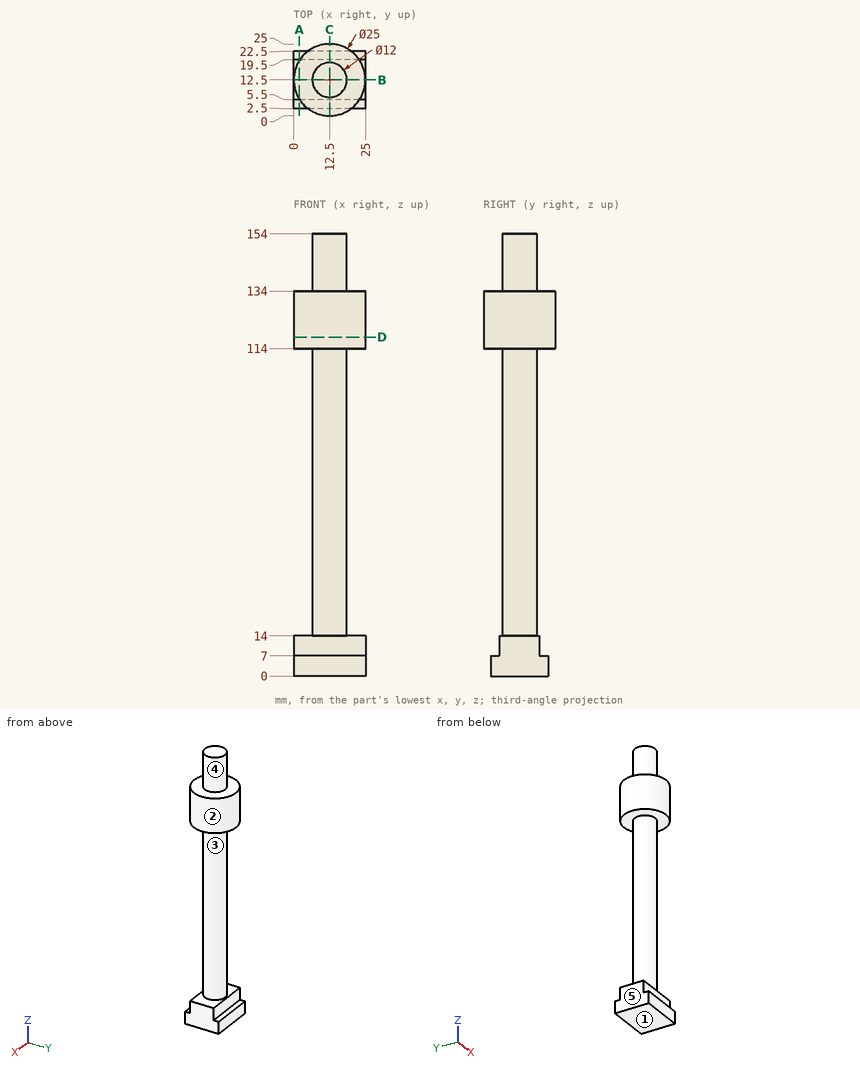
Can you work these out from the drawing? Everything is in mm from the part's minimum corner. A direction names the side the tool comes from. Round coordinates to 2 decimals unless told otherwise and drop trailing zeros. Loops run counter-clockwise (first coordinate to the right, second up) from the corner with the lowest first, then second, coordinate; pieces in that order, holes last. Notation, with made-up numbers: M 38,4 L 46,4 A24 cw 46,40 Z; hole C 83,20.5 d3. An arc over 180 degrees is marked long. Answer in a Markdown table with one row per item.
1. I'm going to push flat-ended pins straight in: pin 1 Ø3 at (x, y) = (19, 20.5) entering from +Z; pin 2 Ø8 at (y, z) = (5, 87.5) entering from +X; pin 3 Ø6 at (x, z) = (17.5, 86.5) entering from -Y. Where does each tip first touch, or does it pass through?
Established:
| item | result |
|---|---|
| pin 1 | z = 134 |
| pin 2 | x = 17.37 |
| pin 3 | y = 6.84 |
2. If we section it at D-D, the plane z = 118: Please give me the cut outline in (x, y).
Established:
| item | result |
|---|---|
| outline | C 12.5,12.5 d25 |
3. Please list where these lines run through material, in increasing order: line 1 (Z direction, x = 7, y = 19.75); line 2 (Z direction, x = 3.25, y = 9.5); line 3 (Y direction, x = 5, z = 117.5). Write a range as from..to.
Established:
| item | result |
|---|---|
| line 1 | 0..7, 114..134 |
| line 2 | 0..14, 114..134 |
| line 3 | 2.5..22.5 |
4. If we section it at B-B, the plane y = 12.5: Please give me the cut outline in (x, z), plus the area to 3 significant figures.
Established:
| item | result |
|---|---|
| outline | M 0,0 L 25,0 L 25,14 L 18.5,14 L 18.5,114 L 25,114 L 25,134 L 18.5,134 L 18.5,154 L 6.5,154 L 6.5,134 L 0,134 L 0,114 L 6.5,114 L 6.5,14 L 0,14 Z |
| area | 2,290 mm² |
5. If we section it at C-C, the plane x = 12.5: Please give me the cut outline in (y, z).
Established:
| item | result |
|---|---|
| outline | M 0,114 L 6.5,114 L 6.5,14 L 5.5,14 L 5.5,7 L 2.5,7 L 2.5,0 L 22.5,0 L 22.5,7 L 19.5,7 L 19.5,14 L 18.5,14 L 18.5,114 L 25,114 L 25,134 L 18.5,134 L 18.5,154 L 6.5,154 L 6.5,134 L 0,134 Z |
6. Thinking about a two-plate mould opening in Z: for the marked faces 1, 2 and 3, which applies, pulls with the +Z half, pulls with the -Z half, needs draft (parallel to the pull), parting line crosses it, or undercut?
Established:
| item | result |
|---|---|
| face 1 | pulls with the -Z half |
| face 2 | needs draft |
| face 3 | undercut |
7. If we section it at A-A, the plane x = 2: Please give me the cut outline in (y, z).
Established:
| item | result |
|---|---|
| outline | M 2.5,0 L 22.5,0 L 22.5,7 L 19.5,7 L 19.5,14 L 5.5,14 L 5.5,7 L 2.5,7 Z; M 5.72,114 L 19.28,114 L 19.28,134 L 5.72,134 Z |
8. On a 3-axis mill with a long thin cutter (end or side, diameter ignored), from which of +Z, -Z, +X, -X, +Y, -Y can I reach the whole of each face in a straight line? I mean the marked faces 4 and 5. Say none if no direction works.
Established:
| item | result |
|---|---|
| face 4 | +Z |
| face 5 | +Z, -Z, -X, +Y, -Y |
